The figure shows three views and two pictorial views of one solid part (mm, origin at its lowest corner). Answer the questions. Coordinates: 2 decimals unless noted, no trailing zeros. Order: outer loops, then holes, each group sorted by start corner. A loop starts at its lowest first (then second) coordinate and runs counter-clockwise, first axis right, second up. Notation, with made-up numbers: (77.25, 52.25) - (117.25, 52.25) arc R28 cw to (117.25, 80.25) - close; hole circle Ø8 at (80.25, 35.25). An arc over 180 degrees is marked (long way). Use one line per item in the form item = value. Start each with the question number.
Item 1: Section C-C, the plane y = 1 is taken. Write down the section's boundary in (x, z) (1 decimal), and give its area (3 significant figures).
Item 2: Consider line 1 along Z through (x, y) = (60.96, 0.75); line 2 along X through (y, z) = (0.8, 2.5); line 3 along X through (y, z) = (0.75, 16.51). Determine where each line is inside the solid, lowest interval first. Write a range as [from, to].
Item 3: Section D-D, the plane x = 83 is taken. Write down the section's boundary in (y, z), and give its area (3 significant figures).
Item 4: Section A-A, the plane x = 60.96 is taken. Write down the section's boundary in (y, z), and give its area (3 significant figures).
Item 5: Section B-B, the plane z = 3 is taken. Write down the section's boundary in (x, y), and give its area (3 significant figures).
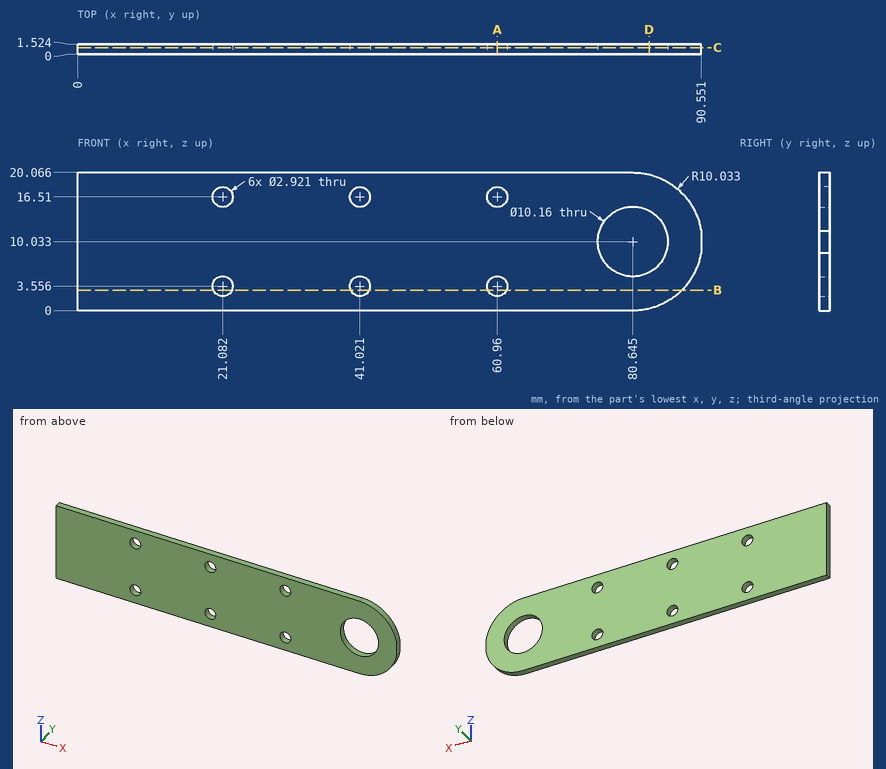
Response:
q1.outline = (0, 0) - (80.6, 0) arc R10 ccw to (90.6, 8.4) - (90.6, 11.6) arc R10 ccw to (80.6, 20.1) - (0, 20.1) - close; hole circle Ø2.9 at (21.1, 3.6); hole circle Ø2.9 at (21.1, 16.5); hole circle Ø2.9 at (41, 3.6); hole circle Ø2.9 at (41, 16.5); hole circle Ø2.9 at (61, 3.6); hole circle Ø2.9 at (61, 16.5); hole circle Ø10.2 at (80.6, 10)
q1.area = 1,650 mm2
q2.line_1 = [0, 2.1], [5.02, 15.05], [17.97, 20.07]
q2.line_2 = [0, 20.07], [22.09, 40.01], [42.03, 59.95], [61.97, 87.27]
q2.line_3 = [0, 19.62], [22.54, 39.56], [42.48, 59.5], [62.42, 88.31]
q3.outline = (0, 0.28) - (1.52, 0.28) - (1.52, 5.53) - (0, 5.53) - close; (0, 14.53) - (1.52, 14.53) - (1.52, 19.79) - (0, 19.79) - close
q3.area = 16.0 mm2
q4.outline = (0, 0) - (1.52, 0) - (1.52, 2.1) - (0, 2.1) - close; (0, 5.02) - (1.52, 5.02) - (1.52, 15.05) - (0, 15.05) - close; (0, 17.97) - (1.52, 17.97) - (1.52, 20.07) - (0, 20.07) - close
q4.area = 21.7 mm2
q5.outline = (0, 0) - (19.73, 0) - (19.73, 1.52) - (0, 1.52) - close; (22.43, 0) - (39.67, 0) - (39.67, 1.52) - (22.43, 1.52) - close; (42.37, 0) - (59.61, 0) - (59.61, 1.52) - (42.37, 1.52) - close; (62.31, 0) - (87.8, 0) - (87.8, 1.52) - (62.31, 1.52) - close
q5.area = 121 mm2
